Can you work these out from the model? Positions are in its coordinate system, mm. Face numbers are marked on the shaded views. A direction names the side the tool comes from. Give positions to 0.01 mm unless a question says otherwise; leave off trailing zeros. Order: outer loops, then holes, each group sorted by start corner. A loop starts at its lowest first (then second) coordinate and runs counter-clockwise, first axis right, second up. Notation, with made-up numbers: (-9.5, 88) - (47.5, 88) arc R31 cw to (47.5, 119) - close; hole circle Ø5 at (-29.5, 31.25). An arc over 180 degrees is marked (long way). Answer as CSV lines item,"result".
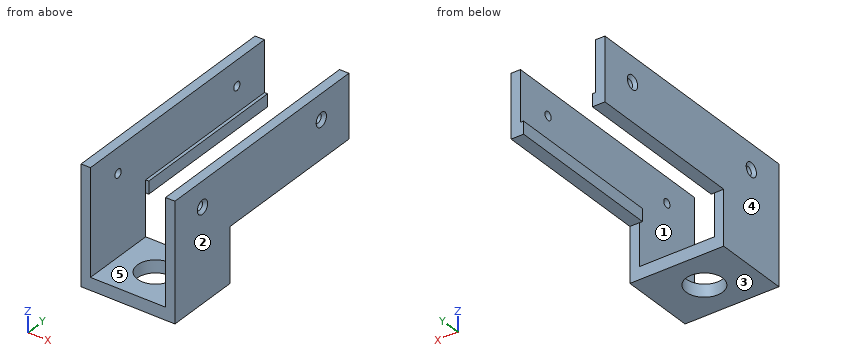
```python
from build123d import *

# Parameters (mm, degrees)
BOSS_EXTRUDE1_DEPTH                            = 38.1
SKETCH7_R                                      = 9.2075
CUT_EXTRUDE2_DEPTH                             = 38.1
SKETCH8_W                                      = 4.7625
SKETCH8_H                                      = 25.654
BOSS_EXTRUDE2_DEPTH                            = 82.042
CSK_FOR_6_FLAT_HEAD_MACHINE_SCREW1_D           = 4.3053
CSK_FOR_6_FLAT_HEAD_MACHINE_SCREW1_DEPTH       = 4.7625
CSK_FOR_6_FLAT_HEAD_MACHINE_SCREW1_CSINK_D     = 7.0866
CSK_FOR_6_FLAT_HEAD_MACHINE_SCREW1_CSINK_ANGLE = 82
CSK_FOR_6_FLAT_HEAD_MACHINE_SCREW2_D           = 4.3053
CSK_FOR_6_FLAT_HEAD_MACHINE_SCREW2_CSINK_D     = 7.0866
CSK_FOR_6_FLAT_HEAD_MACHINE_SCREW2_CSINK_ANGLE = 82
SKETCH9_W                                      = 6.35
SKETCH9_H                                      = 82.042
BOSS_EXTRUDE3_DEPTH                            = 6.35


with BuildPart() as part:
    # Sketch1 → Boss-Extrude1 (new body)
    with BuildSketch(Plane(origin=(0, 0, 0), x_dir=(1, 0, 0), z_dir=(0, 1, 0))):
        Polygon((0, 0), (0, 59.69), (47.625, 59.69), (47.625, 0), (42.8625, 0), (42.8625, 53.34), (4.7625, 53.34), (4.7625, 0), align=None)
    extrude(amount=BOSS_EXTRUDE1_DEPTH)

    # Sketch7 → Cut-Extrude2 (cut)
    with BuildSketch(Plane(origin=(0, 0, -59.69), x_dir=(-1, 0, 0), z_dir=(0, 0, -1))):
        with Locations((-23.8125, 19.05)):
            Circle(SKETCH7_R)
    extrude(amount=-CUT_EXTRUDE2_DEPTH, mode=Mode.SUBTRACT)

    # Sketch8 → Boss-Extrude2 (add)
    with BuildSketch(Plane(origin=(0, 38.1, 0), x_dir=(1, 0, 0), z_dir=(0, 1, 0))):
        with Locations((2.38125, 12.827)):
            Rectangle(SKETCH8_W, SKETCH8_H)
        with Locations((45.24375, 12.827)):
            Rectangle(SKETCH8_W, SKETCH8_H)
    extrude(amount=BOSS_EXTRUDE2_DEPTH)

    # CSK for #6 Flat Head Machine Screw1
    with Locations(Plane.ZY):
        with Locations((-12.7, 19.05), (-12.7, 101.092)):
            CounterSinkHole(CSK_FOR_6_FLAT_HEAD_MACHINE_SCREW1_D / 2, CSK_FOR_6_FLAT_HEAD_MACHINE_SCREW1_CSINK_D / 2, depth=CSK_FOR_6_FLAT_HEAD_MACHINE_SCREW1_DEPTH, counter_sink_angle=CSK_FOR_6_FLAT_HEAD_MACHINE_SCREW1_CSINK_ANGLE)

    # CSK for #6 Flat Head Machine Screw2 (through all)
    with Locations(Plane(origin=(47.625, 0, 0), x_dir=(0, 0, -1), z_dir=(1, 0, 0))):
        with Locations((12.7, 19.05), (12.7, 101.092)):
            CounterSinkHole(CSK_FOR_6_FLAT_HEAD_MACHINE_SCREW2_D / 2, CSK_FOR_6_FLAT_HEAD_MACHINE_SCREW2_CSINK_D / 2, counter_sink_angle=CSK_FOR_6_FLAT_HEAD_MACHINE_SCREW2_CSINK_ANGLE)

    # Sketch9 → Boss-Extrude3 (add)
    with BuildSketch(Plane(origin=(0, 0, -25.654), x_dir=(-1, 0, 0), z_dir=(0, 0, -1))):
        with Locations((-3.175, 79.121)):
            Rectangle(SKETCH9_W, SKETCH9_H)
        with Locations((-44.45, 79.121)):
            Rectangle(SKETCH9_W, SKETCH9_H)
    extrude(amount=BOSS_EXTRUDE3_DEPTH)


solid = part.part
```
1) I want a section at D-D on z = -12.7. Count the separate pieces of the cut face and the enclosed holes in it, plus the area to 3 significant figures.
Answer block:
separate pieces,"6"
enclosed holes,"0"
area,"1,050 mm2"
2) If we mould it in two halves opening along X, with no side actions, what happens to the marked faces 1, 2 and 3? For each: +X half, -X half, draft (parallel to the pull), parting line (faces both ways), or undercut.
Answer block:
face 1,"undercut"
face 2,"+X half"
face 3,"draft"
3) I'm going to push flat-ended pins straight in: P1, Ø5.5, axis at y = 101.092, z = -12.7, coming from the -X side; P2, Ø1.3, axis at x = 5.5, y = 76, coming from the +Z side; P3, Ø1.9, axis at x = 3.5, y = 94.5, coming from the -Z side. Where does each tip first touch, or does it pass through?
Answer block:
P1,"x = 0.91"
P2,"z = -25.65"
P3,"z = -32"
4) I need wall thicknesses on line 1 along Y through (x, z) = (3.55, -12.7); line 2 along Z through (x, y) = (43.75, 19.05); line 3 along X through (y, z) = (7.5, -33.5) (1 decimal). Which ranges of each line are inside material? Lowest first, please. Write a range as [from, to].
Answer block:
line 1,"[0, 16.9], [21.2, 98.94], [103.24, 120.14]"
line 2,"[-59.69, -14.85], [-10.55, 0]"
line 3,"[0, 4.8], [42.9, 47.6]"
5) I want a section at B-B on y = 19.05. Write out the boundary of the cut face in (x, z) (1 decimal).
Answer block:
outline,"(0, -59.7) - (14.6, -59.7) - (14.6, -53.3) - (4.8, -53.3) - (4.8, -14.9) - (1.6, -14.9) - (0, -16.2) - close; (0, -9.2) - (1.6, -10.5) - (4.8, -10.5) - (4.8, 0) - (0, 0) - close; (33, -59.7) - (47.6, -59.7) - (47.6, -16.2) - (46, -14.9) - (42.9, -14.9) - (42.9, -53.3) - (33, -53.3) - close; (42.9, -10.5) - (46, -10.5) - (47.6, -9.2) - (47.6, 0) - (42.9, 0) - close"
6) Which directions (+Z, -Z, +X, -X, +Y, -Y) give clear straight access to the entire face, cutting with the end or side of a thin tool? Please do the marked faces 4 and 5.
Answer block:
face 4,"+Z, -Z, -X, +Y, -Y"
face 5,"+Z, +Y, -Y"
